Geometry check sheet. Reference: drawing and pictorial views, mm from the part's lowest x, y, z. Round coordinates to 2 decimals unless told otherwise and drop trailing zeros. Write each loop counter-clockwise with the first axis right and the second up, starting at its lowest first coordinate (ties: lowest second). Pieces come first, ordered by that corner, then holes.
Item 1: Section check A-A, the plane z = 101. Record the cut outline in (x, y), plus the area to 3 significant figures.
Item 2: Depth check by flat-ended pin: pin 1 (10 mm diameter, centred on x = 253.5, z = 53.5, fed in from -Y). Enter the tip coordinate at first touch or a pass-through.
Item 3: Material ranges on line 1 along Z through (x, y) = (114, 24.5); line 2 along Y through (x, z) = (21.5, 100.5); line 3 along X through (y, z) = (98, 101), recorded low to high.
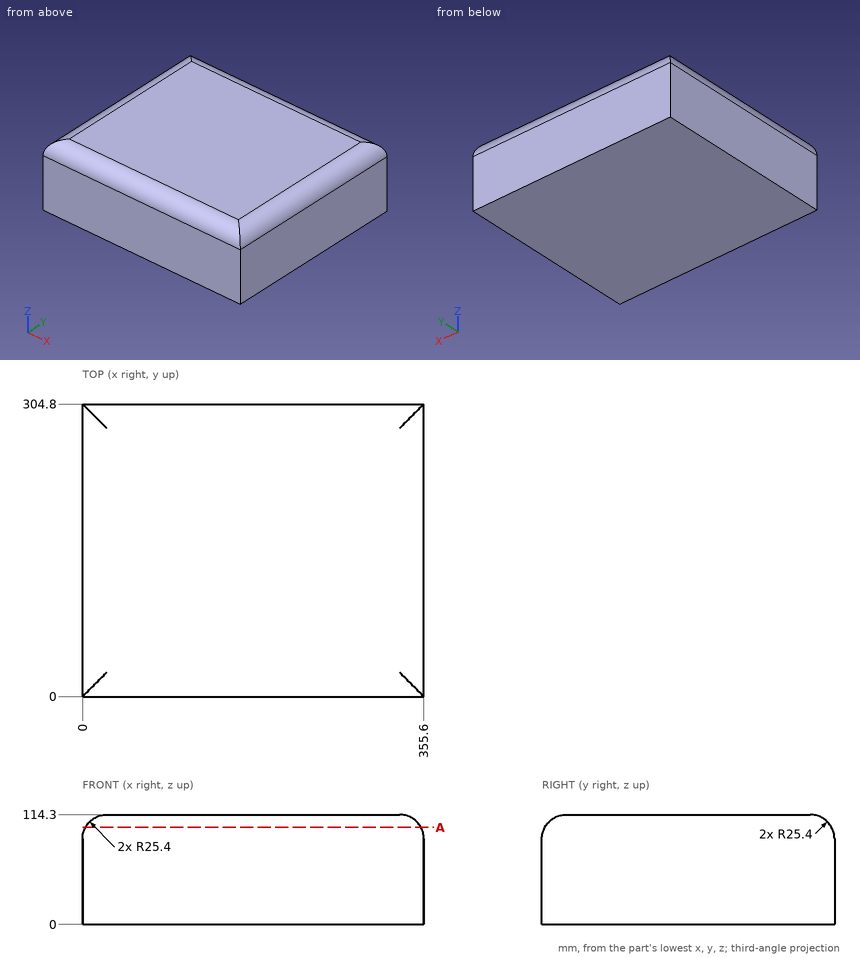
Values found:
1. outline: (3.07, 3.07) - (352.53, 3.07) - (352.53, 301.73) - (3.07, 301.73) - close
1. area: 104,000 mm2
2. pin 1: stops at y = 0
3. line 1: z = 0 to 114.28
3. line 2: y = 2.8 to 302
3. line 3: x = 3.07 to 352.53
